Autodesk Inventor part; units mm, degrees
ref_plane "YZ Plane" through (0, 0, 0) normal (1, 0, 0) x (0, 1, 0)
ref_plane "XZ Plane" through (0, 0, 0) normal (0, 1, 0) x (-1, 0, 0)
ref_plane "XY Plane" through (0, 0, 0) normal (0, 0, 1) x (1, 0, 0)
sketch "Sketch1" plane through (0, 0, 0) normal (0, 0, 1) x (1, 0, 0)
  circle A0 centre (0, 0) radius 1.5
  dimension "d0" = 3
extrude "Extrusion1" add sketch "Sketch1" along normal blind 8
sketch "Sketch2" plane through (0, 0, 0) normal (0, 0, -1) x (-1, 0, 0)
  circle A0 centre (0, 0) radius 1.5
  circle A1 centre (0, 0) radius 2.25
  dimension "d3" = 4.5
extrude "Extrusion2" add sketch "Sketch2" along normal blind 3 contours A0 | A1
sketch "Sketch3" plane through (0, 0, -3) normal (0, 0, -1) x (-1, 0, 0)
  circle A0 centre (0, 0) radius 2.25
  line L0 (-0.7217, 1.25) -> (0.7217, 1.25)
  line L1 (0.7217, 1.25) -> (1.4434, 0)
  line L2 (1.4434, 0) -> (0.7217, -1.25)
  line L3 (0.7217, -1.25) -> (-0.7217, -1.25)
  line L4 (-0.7217, -1.25) -> (-1.4434, 0)
  line L5 (-1.4434, 0) -> (-0.7217, 1.25)
  dimension "d6" = 2.5
extrude "Extrusion3" cut sketch "Sketch3" against normal blind 1.5 contours L0 L1 L2 L3 L4 L5
thread "Thread1"
chamfer "Chamfer1" distance 0.508 angle 45 1 edges at (-1.5, 0, 8)
chamfer "Chamfer2" distance 0.25 angle 45 1 edges at (2.25, 0, -3)
properties part number "M3 SHCS x8" material "Steel"
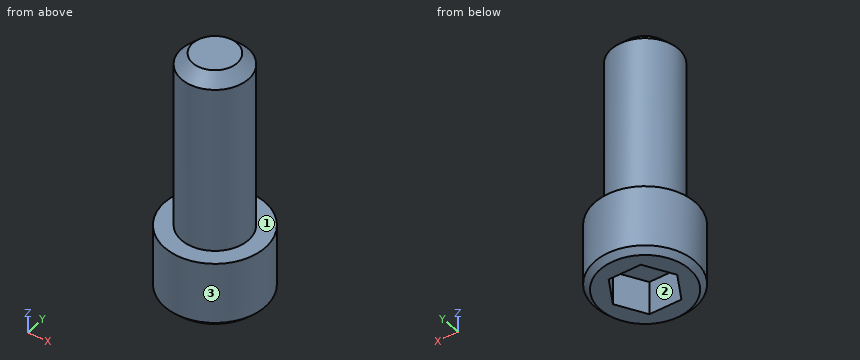
Input: part model. Units: mm. Frame: model coordinates. Face numbers are marked on the shaded views. A direction names the side the tool comes from. Coordinates: 2 decimals unless noted, no trailing zeros. Loops run counter-clockwise (first coordinate to the right, second up) from the corner with the lowest first, then second, coordinate; pieces in that order, holes last.
(1) Section A-A on x = 0. Return the cut outline in (y, z).
(2) Material intervals for probe 1 along Z at (x, y) = (-0.25, 0.15); probe 2 along Y at (x, z) = (0, 6.25); probe 3 along X at (y, z) = (0.4, 2.25), sorted ascending.
(3) Set-up query: the marked faces 1, 2 and 3. Return all of +Z, -Z, +X, -X, +Y, -Y with unobstructed straight access to the full face (end or side cutting, diameter ignored); none if empty.
(4) First-contact query: pin 1 Ø1 at (x, z) = (0.5, 4.5) entering from +Y; pin 2 Ø0.8 at (x, y) = (-0.5, -0.5) entering from -Z. Flat tips, straight axial feed; report the tip coordinate or a pass-through.
(5) Section B-B on z = 5.5. Return the cut outline in (x, y), then the cut area to 3 significant figures.
Data:
1. outline: (-2.25, -2.75) - (-2, -3) - (-1.25, -3) - (-1.25, -1.5) - (1.25, -1.5) - (1.25, -3) - (2, -3) - (2.25, -2.75) - (2.25, 0) - (1.5, 0) - (1.5, 7.49) - (0.99, 8) - (-0.99, 8) - (-1.5, 7.49) - (-1.5, 0) - (-2.25, 0) - close
2. probe 1: z = -1.5 to 8
2. probe 2: y = -1.5 to 1.5
2. probe 3: x = -1.45 to 1.45
3. face 1: +Z
3. face 2: -Z
3. face 3: +Z, -Z
4. pin 1: stops at y = 1.5
4. pin 2: stops at z = -1.5
5. outline: circle Ø3 at (0, 0)
5. area: 7.07 mm2
